from build123d import *

# Parameters (mm, degrees)
SKETCH1_W = 1.5
SKETCH1_H = 4
FILLET1_R = 0.25


with BuildPart() as part:
    # Sketch1 → Revolve1 (revolve)
    with BuildSketch(Plane.XY):
        with Locations((-19.25, 0)):
            Rectangle(SKETCH1_W, SKETCH1_H)
    revolve(axis=Axis((0, 0, 0), (0, 1, 0)))

    # Fillet1
    fillet1_edges = [part.edges().sort_by_distance(p)[0] for p in [
        (20, 2, 0),
        (18.5, 2, 0),
        (18.5, -2, 0),
        (20, -2, 0),
    ]]
    fillet(fillet1_edges, radius=FILLET1_R)


solid = part.part
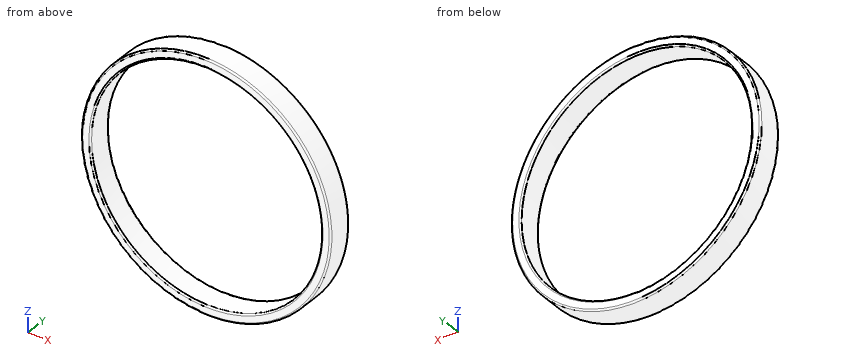
Here's how the part is built. I have some questions about the finished solid (model axes, mm). Give positions to 0.01 mm unless a question says otherwise; leave off trailing zeros. Loops run counter-clockwise (first coordinate to the right, second up) from the corner with the lowest first, then second, coordinate; pieces in that order, holes last. Notation, with made-up numbers: (-17, -17) -> (7, -17) arc R27 cw to (7, 14) -> close; hole circle Ø6 at (-11.5, -20). An arc over 180 degrees is marked (long way). Answer as a JSON object with one key per item and string values. Group by question number.
Item 1: Imagine slicing it at C-C on y = 0.5. Write out the boundary of the cut face in (x, z).
Item 2: I need wall thicknesses on L1, parallel to Z at x = 0, y = 0.5; L2, parallel to X at y = 1.55, z = 7 (3 decimals); L3, parallel to X at y = 0.25, z = 14. Which ranges of each line are inside material? Lowest first, please.
Item 3: Will this pin go through, and if not, where does the flat tip stop? pin 1 (12 mm diameter, centred on x = -8, z = 4, fed in from +Y).
Item 4: Imagine slicing it at A-A on z = 0. Write out the boundary of the cut face in (x, y), then the cut area to 3 significant figures.
Item 5: Imagine slicing it at B-B on x = 0. Write out the boundary of the cut face in (y, z), then the cut area to 3 significant figures.
Answer list:
{
 "1": {"outline": "circle Ø40 at (0, 0); hole circle Ø37 at (0, 0)"},
 "2": {"L1": "z = -20 to -18.5, 18.5 to 20", "L2": "x = -18.735 to -17.125, 17.125 to 18.735", "L3": "x = -14.28 to -12.09, 12.09 to 14.28"},
 "3": {"pin 1": "passes through"},
 "4": {"outline": "(-20, -1.75) arc R0.25 ccw to (-19.75, -2) -> (-18.75, -2) arc R0.25 ccw to (-18.5, -1.75) -> (-18.5, 1.75) arc R0.25 ccw to (-18.75, 2) -> (-19.75, 2) arc R0.25 ccw to (-20, 1.75) -> close; (18.5, -1.75) arc R0.25 ccw to (18.75, -2) -> (19.75, -2) arc R0.25 ccw to (20, -1.75) -> (20, 1.75) arc R0.25 ccw to (19.75, 2) -> (18.75, 2) arc R0.25 ccw to (18.5, 1.75) -> close", "area": "11.9 mm2"},
 "5": {"outline": "(-2, -19.75) arc R0.25 ccw to (-1.75, -20) -> (1.75, -20) arc R0.25 ccw to (2, -19.75) -> (2, -18.75) arc R0.25 ccw to (1.75, -18.5) -> (-1.75, -18.5) arc R0.25 ccw to (-2, -18.75) -> close; (-2, 18.75) arc R0.25 ccw to (-1.75, 18.5) -> (1.75, 18.5) arc R0.25 ccw to (2, 18.75) -> (2, 19.75) arc R0.25 ccw to (1.75, 20) -> (-1.75, 20) arc R0.25 ccw to (-2, 19.75) -> close", "area": "11.9 mm2"}
}
